Solid Edge part; units mm, degrees
sketch "Sketch1" plane through (0, 0, 0) normal (0, 0, 1) x (1, 0, 0)
  line L0 (25.3811, -4.212) -> (25.3811, 0.788)
  line L1 (25.3811, 0.788) -> (0.3811, 0.788)
  line L2 (0.3811, 0.788) -> (0.3811, -4.212)
  line L3 (0.3811, -4.212) -> (25.3811, -4.212)
extrude "Protrusion1" add sketch "Sketch1" along normal blind 25
sketch "Sketch2" plane through (0.3811, -1.712, 12.5) normal (-1, 0, 0) x (0, 0, 1)
  line L0 (8.5, -2.5) -> (8.5, 2.5)
  line L1 (8.5, 2.5) -> (-12.5, 2.5)
  line L2 (-12.5, 2.5) -> (-12.5, -2.5)
  line L3 (-12.5, -2.5) -> (8.5, -2.5)
extrude "ExtrudedProtrusion_4" add sketch "Sketch2" along normal blind 3
sketch "Sketch3" plane through (25.3811, -1.712, 12.5) normal (1, 0, 0) x (0, 0, -1)
  line L0 (-8.5, -2.5) -> (-8.5, 2.5)
  line L1 (-8.5, 2.5) -> (12.5, 2.5)
  line L2 (12.5, 2.5) -> (12.5, -2.5)
  line L3 (12.5, -2.5) -> (-8.5, -2.5)
extrude "ExtrudedProtrusion_5" add sketch "Sketch3" along normal blind 3
Work out the finished part from the listing and answer in its coordinate system (mm). A direction names the side the tool comes from. Coordinates: 2 decimals unless noted, no trailing zeros. Loops run counter-clockwise (first coordinate to the right, second up) from the corner with the lowest first, then second, coordinate; pieces in that order, holes last. Notation, with made-up numbers: (72.5, -13) -> (93.5, -13) arc R19 cw to (93.5, 5) -> close; hole circle Ø4 at (10, 44). An arc over 180 degrees is marked (long way). Write each question's results on one line, items separated by ' | '. Start each with the question number.
1) Find section B-B on z = 23. Determine the outline of the cut face in (x, y), then the cut area to 3 significant figures.
2) For faces 1 (the flat face through (25.381, -2, 23)), 2 (the flat face through (-2.619, -2, 11)), 3 (the flat face through (0.381, -2, 23)), determine the directions among +Z, -Z, +X, -X, +Y, -Y from which every point of the face is accessible in a straight line to the end or side of a thin tool.
3) Find section A-A on y = -0.35. Determine the outline of the cut face in (x, z), then the cut area to 3 significant figures.
4) Flat-ended cylindrical pins translate along their axes: P1, Ø1.5, axis at x = -1, y = -1.5, coming from the +Z side; P2, Ø1.2, axis at y = -0.5, z = 24, coming from the +X side. Find the tip coordinate at first contact, or state that the pin passes through.
5) Consider line 1 along X through (y, z) = (-2.1, 24); line 2 along Z through (x, y) = (26, -2.4). Determine where each line is inside the solid, lowest interval first.
Response values:
1) outline: (0.38, -4.21) -> (25.38, -4.21) -> (25.38, 0.79) -> (0.38, 0.79) -> close | area: 125 mm^2
2) face 1: +Z, +X, +Y, -Y | face 2: +Z, -Z, -X, +Y, -Y | face 3: +Z, -X, +Y, -Y
3) outline: (-2.62, 0) -> (28.38, 0) -> (28.38, 21) -> (25.38, 21) -> (25.38, 25) -> (0.38, 25) -> (0.38, 21) -> (-2.62, 21) -> close | area: 751 mm^2
4) P1: stops at z = 21 | P2: stops at x = 25.38
5) line 1: x = 0.38 to 25.38 | line 2: z = 0 to 21
